Autodesk Inventor part; units mm, degrees
ref_plane "YZ Plane" through (0, 0, 0) normal (1, 0, 0) x (0, 1, 0)
ref_plane "XZ Plane" through (0, 0, 0) normal (0, 1, 0) x (-1, 0, 0)
ref_plane "XY Plane" through (0, 0, 0) normal (0, 0, 1) x (1, 0, 0)
sketch "Sketch1" plane through (0, 0, 0) normal (0, 1, 0) x (-1, 0, 0)
  line L0 (90, -50) -> (-90, -50)
  line L1 (-90, -50) -> (-90, 50)
  line L2 (-90, 50) -> (90, 50)
  line L3 (90, 50) -> (90, -50)
  line L4 (0, 0) -> (0, -16.1308) construction
  line L5 (0, 0) -> (18.4922, 0) construction
  dimension "d1" = 100
  dimension "d2" = 180
extrude "Extrusion1" add sketch "Sketch1" along normal blind 2.2
sketch "Sketch2" plane through (0, 2.2, 0) normal (0, 1, 0) x (1, 0, 0)
  line L0 (-90, -50) -> (90, -50)
  line L1 (90, -50) -> (90, 50)
  line L2 (90, -50) -> (90, -30)
  line L3 (90, -30) -> (55.6, -30)
  line L4 (55.6, -30) -> (55.6, -50)
  line L5 (55.6, -50) -> (90, -50)
  line L6 (90, -40) -> (55.6, -40) construction
  circle A0 centre (78.8, -40) radius 2.15
  circle A1 centre (72.8, -40) radius 2.15
  circle A2 centre (66.8, -40) radius 2.15
  line L7 (72.8, -40) -> (72.8, -30) construction
  circle A3 centre (72.8, -34) radius 2.15
  circle A4 centre (72.8, -46) radius 2.15
  circle A5 centre (72.8, -40) radius 2.15
  line L8 (0, 0) -> (96.2626, 0) construction
  line L9 (90, 50) -> (90, 30)
  line L10 (90, 30) -> (55.6, 30)
  line L11 (55.6, 30) -> (55.6, 50)
  line L12 (55.6, 50) -> (90, 50)
  line L13 (90, 40) -> (55.6, 40) construction
  circle A6 centre (78.8, 40) radius 2.15
  circle A7 centre (72.8, 40) radius 2.15
  circle A8 centre (66.8, 40) radius 2.15
  line L14 (72.8, 40) -> (72.8, 30) construction
  circle A9 centre (72.8, 34) radius 2.15
  circle A10 centre (72.8, 46) radius 2.15
  circle A11 centre (72.8, 40) radius 2.15
  line L15 (90, 50) -> (-90, 50)
  line L16 (-90, 50) -> (-90, -50)
  line L17 (-48, 40) -> (-72, 40)
  line L18 (-72, 40) -> (-72, 50)
  line L19 (-72, 50) -> (-48, 50)
  line L20 (-48, 50) -> (-48, 40)
  line L21 (-74.3246, 46.5) -> (-4.1674, 46.5) construction
  line L22 (-60, 53.3324) -> (-60, 32.9187) construction
  circle A12 centre (-60, 37.5) radius 2.15
  line L23 (-68.3246, 46.5) -> (1.8326, 46.5) construction
  circle A13 centre (-54, 37.5) radius 2.15
  circle A14 centre (-66, 37.5) radius 2.15
  line L24 (-8.0003, 43.25) -> (-83.9137, 43.25) construction
  circle A15 centre (-78, 43.25) radius 2.15
  circle A16 centre (-84, 43.25) radius 2.15
  circle A17 centre (-42, 43.25) radius 2.15
  circle A18 centre (-36, 43.25) radius 2.15
  line L25 (-48, -40) -> (-72, -40)
  line L26 (-72, -40) -> (-72, -50)
  line L27 (-72, -50) -> (-48, -50)
  line L28 (-48, -50) -> (-48, -40)
  line L29 (-74.3246, -46.5) -> (-4.1674, -46.5) construction
  line L30 (-60, -53.3324) -> (-60, -32.9187) construction
  circle A19 centre (-60, -37.5) radius 2.15
  circle A20 centre (-54, -37.5) radius 2.15
  circle A21 centre (-66, -37.5) radius 2.15
  line L31 (-8.0003, -43.25) -> (-83.9137, -43.25) construction
  circle A22 centre (-78, -43.25) radius 2.15
  circle A23 centre (-84, -43.25) radius 2.15
  circle A24 centre (-36, -43.25) radius 2.15
  circle A25 centre (-42, -43.25) radius 2.15
  circle A26 centre (-60, 37.5) radius 2.5 construction
  dimension "d13" = 20
  dimension "d14" = 34.4
  dimension "d15" = 4.3
  dimension "d16" = 6
  dimension "d17" = 6
  dimension "d18" = 6
  dimension "d27" = 24
  dimension "d28" = 10
  dimension "d29" = 18
  dimension "d31" = 4.3
  dimension "d34" = 6
  dimension "d41" = 6
  dimension "d46" = 6.5
  dimension "d48" = 4.3
  dimension "d49" = 6
  dimension "d52" = 6
  dimension "d60" = 5
extrude "Holes" cut sketch "Sketch2" against normal through all contours A0 | A1 | A2 | A3 | A4 | A6 | A7 | A8 | A9 | A10 | A12 | A13 | A14 | A15 | A16 | A17 | A18 | A19 | A20 | A21 | A22 | A23 | A24 | A25
sketch "Sketch3" plane through (0, 2.2, 0) normal (0, 1, 0) x (1, 0, 0)
  line L0 (33.5, 13.5) -> (-33.5, 13.5) construction
  line L1 (-33.5, 13.5) -> (-33.5, -13.5) construction
  line L2 (-33.5, -13.5) -> (33.5, -13.5) construction
  line L3 (33.5, -13.5) -> (33.5, 13.5) construction
  line L4 (0, 0) -> (39.98, 0) construction
  line L5 (0, 0) -> (0, 21.0122) construction
  circle A0 centre (30, 9) radius 2.15
  circle A1 centre (30, -9) radius 2.15
  circle A2 centre (-30, 9) radius 2.15
  circle A3 centre (-30, -9) radius 2.15
  line L6 (33.5, 7.5) -> (43.5, 7.5)
  line L7 (43.5, 7.5) -> (43.5, -7.5)
  line L8 (43.5, -7.5) -> (33.5, -7.5)
  line L9 (33.5, -7.5) -> (33.5, 7.5)
  dimension "d61" = 67
  dimension "d62" = 27
  dimension "d63" = 4.3
  dimension "d64" = 3.5
  dimension "d65" = 4.5
  dimension "d68" = 10
  dimension "d69" = 15
extrude "Extrusion4" cut sketch "Sketch3" against normal through all
fillet "Fillet1" radius 2 4 edges at (33.5, 1.1, -7.5) (43.5, 1.1, -7.5) (43.5, 1.1, 7.5) (33.5, 1.1, 7.5)
ref_plane "Work Plane1" through (0, 0, 50) normal (1, 0, 0) x (0, 0, -1)
split "Split1" plane through (0, 0, 50) removes the side toward (1, 0, 0)
sketch "Sketch4" plane through (0, 2.2, 0) normal (0, 1, 0) x (1, 0, 0)
  line L0 (0, 50) -> (-90, 50)
  line L1 (-90, -50) -> (0, -50)
  line L2 (0, 50) -> (-5, 50) construction
  line L3 (-5, 50) -> (-5, -50) construction
  line L4 (-5, -50) -> (0, -50) construction
  line L5 (0, -50) -> (0, 50) construction
  line L6 (0, 0) -> (-126.431, 0) construction
  circle A0 centre (-5, 37.5) radius 1.3
  circle A1 centre (-5, 25) radius 1.3
  circle A2 centre (-5, -37.5) radius 1.3
  circle A3 centre (-5, -25) radius 1.3
  dimension "d71" = 5
  dimension "d72" = 2.6
  dimension "d73" = 12.5
  dimension "d76" = 12.5
extrude "Extrusion5" cut sketch "Sketch4" against normal through all
equation "\"d1\" = BodyWidth"
equation "\"d2\" = BodyLength"
equation "\"d3\" = Depth"
equation "\"d15\" = Holes"
equation "\"d27\" = MotorWidth"
equation "\"d31\" = Holes"
equation "\"d57\" = Depth"
equation "\"d73\" = 0.125 * BodyWidth"
equation "\"d76\" = 0.125 * BodyWidth"
equation "\"BodyWidth\" = 100"
equation "\"BodyLength\" = 180"
equation "\"Holes\" = 4.3"
equation "\"Depth\" = 2.2"
equation "\"d20\" = 4.3"
equation "\"MotorWidth\" = 24"
properties part number "BodyFront"
The model under review builds one solid part; all positions refer to its coordinate system, in mm. Round coordinates to 2 decimals unless told otherwise and drop trailing zeros. Write each loop counter-clockwise with the first axis right and the second up, starting at its lowest first coordinate (ties: lowest second). Pieces come first, ordered by that corner, then holes.
(1) Wall thickness on L1, parallel to Z at x = -60, y = 1; L2, parallel to X at y = 0.8, z = 37.5; L3, parallel to X at y = 1.2, z = 43.25: over which ranges is each line inside the solid? List them lowest first.
(2) Insertion check: pin 1 (7 mm diameter, centred on x = -30, z = 9, fed in from +Y); pin 2 (3.5 mm diameter, centred on x = -78, z = 43.25, fed in from +Y). Each pin has a flat end and moves straight along its axis. Give the tip position at first contact, or say it passes through.
(3) We need section C-C on z = 43.25. Give the boundary of the cut face in (x, y), and give its area (3 significant figures).
(4) We need section A-A on z = -9. Give the boundary of the cut face in (x, y), and give its area (3 significant figures).
(5) We need section D-D on y = 1.2. Give the number of separate pieces and of enclosed holes in the cut face, and give its area (3 significant figures).
(6) We need section B-B on x = -66. Give the boundary of the cut face in (y, z), and give its area (3 significant figures).
(7) Mouldability with a two-part tool opening along X and no side actions: class faces 1 (the cylindrical face through (-34.84, 1.12, 41.44)), 2 (the flat face through (-44, 1, 50)), 3 (the flat face through (-90, 1, 1)), 4 (the flat face through (0, 1, -1)) as +X half, -X half, draft (parallel to the pull), parting line (faces both ways), or undercut.
Findings below:
1. L1: z = -50 to -39.65, -35.35 to 35.35, 39.65 to 50
1. L2: x = -90 to -68.15, -63.85 to -62.15, -57.85 to -56.15, -51.85 to -6.3, -3.7 to 0
1. L3: x = -90 to -86.15, -81.85 to -80.15, -75.85 to -44.15, -39.85 to -38.15, -33.85 to 0
2. pin 1: stops at y = 2.2
2. pin 2: passes through
3. outline: (-90, 0) - (-86.15, 0) - (-86.15, 2.2) - (-90, 2.2) - close; (-81.85, 0) - (-80.15, 0) - (-80.15, 2.2) - (-81.85, 2.2) - close; (-75.85, 0) - (-44.15, 0) - (-44.15, 2.2) - (-75.85, 2.2) - close; (-39.85, 0) - (-38.15, 0) - (-38.15, 2.2) - (-39.85, 2.2) - close; (-33.85, 0) - (0, 0) - (0, 2.2) - (-33.85, 2.2) - close
3. area: 160 mm2
4. outline: (-90, 0) - (-32.15, 0) - (-32.15, 2.2) - (-90, 2.2) - close; (-27.85, 0) - (0, 0) - (0, 2.2) - (-27.85, 2.2) - close
4. area: 189 mm2
5. separate pieces: 1
5. enclosed holes: 20
5. area: 8,750 mm2
6. outline: (0, -50) - (2.2, -50) - (2.2, -39.65) - (0, -39.65) - close; (0, -35.35) - (2.2, -35.35) - (2.2, 35.35) - (0, 35.35) - close; (0, 39.65) - (2.2, 39.65) - (2.2, 50) - (0, 50) - close
6. area: 201 mm2
7. face 1: undercut
7. face 2: draft
7. face 3: -X half
7. face 4: +X half
